Print and shaded views of the part. All mm, measured from the part's lowest x, y and z. Give positions to 0.01 mm unless a question says otherwise; leave off trailing zeros. Order: outer loops, then holes, each group sorted by start corner. A loop starts at its lowest first (then second) coordinate and runs counter-clockwise, first axis right, second up. Notation, with made-up numbers: (42.5, 31) - (86.5, 31) arc R15 ccw to (86.5, 54) - close; hole circle Ø7 at (82.25, -25.5). An arc over 180 degrees is marked (long way). Answer in a Markdown table with one row per item.
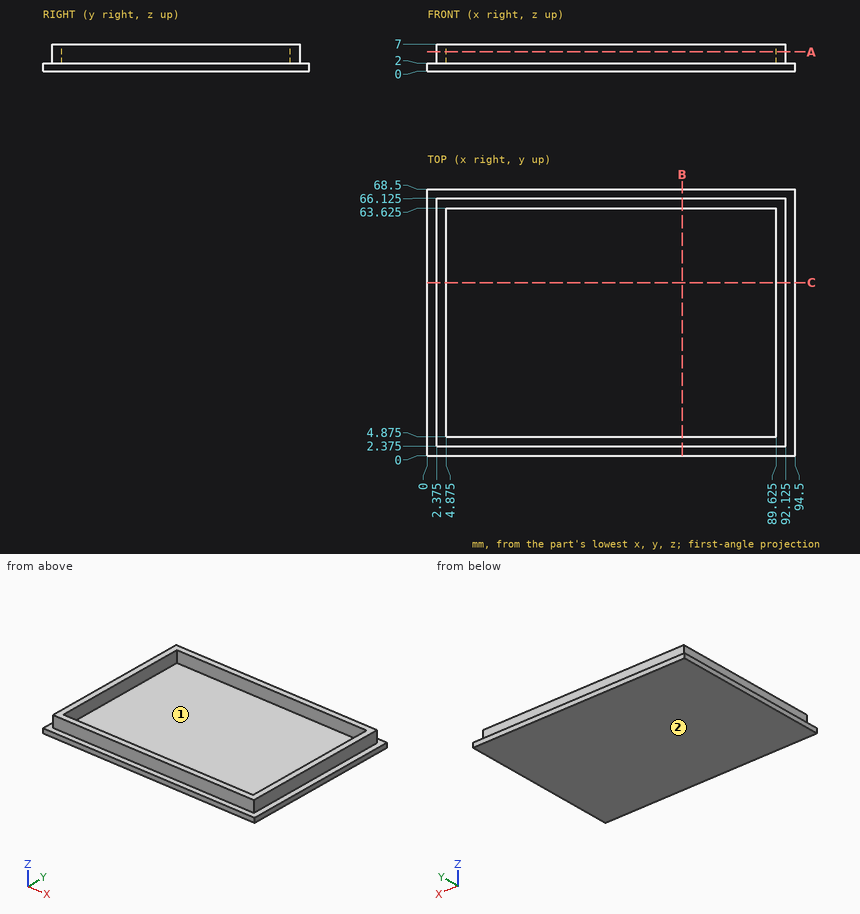
1. Cut at C-C on y = 44.5. Write the cut outline in (x, z) (3 decimals).
Check result:
| item | result |
|---|---|
| outline | (0, 0) - (94.5, 0) - (94.5, 2) - (92.125, 2) - (92.125, 7) - (89.625, 7) - (89.625, 2) - (4.875, 2) - (4.875, 7) - (2.375, 7) - (2.375, 2) - (0, 2) - close |
2. Two-plate mould, pull along Y, no slides. Class the marked faces 1 and 2: +Y half, -Y half, draft (parallel to the pull), parting line (faces both ways), or undercut.
Check result:
| item | result |
|---|---|
| face 1 | undercut |
| face 2 | draft |
3. Probe line 1 (X direction, y = 25.5, z = 4.5) (3 decimals); line 2 (Y direction, x = 45.5, z = 6.5) (3 decimals); line 3 (Z direction, x = 83.5, y = 54.5). List the from-to ranges inside material, lowest first.
Check result:
| item | result |
|---|---|
| line 1 | x = 2.375 to 4.875, 89.625 to 92.125 |
| line 2 | y = 2.375 to 4.875, 63.625 to 66.125 |
| line 3 | z = 0 to 2 |
4. Cut at B-B on x = 65.5. Write the cut outline in (y, z) (3 decimals).
Check result:
| item | result |
|---|---|
| outline | (0, 0) - (68.5, 0) - (68.5, 2) - (66.125, 2) - (66.125, 7) - (63.625, 7) - (63.625, 2) - (4.875, 2) - (4.875, 7) - (2.375, 7) - (2.375, 2) - (0, 2) - close |
5. Drop flat-ended pins along their axis: P1, Ø1.5, axis at x = 45.5, z = 5, coming from the +Y side (3 decimals); P2, Ø2.5, axis at x = 60, z = 4, coming from the -Y side (3 decimals); P3, Ø10, axis at x = 11, y = 43.5, coming from the +Z side. Give the stop position or say it passes through.
Check result:
| item | result |
|---|---|
| P1 | stops at y = 66.125 |
| P2 | stops at y = 2.375 |
| P3 | stops at z = 2 |
6. Cut at A-A on z = 5. Write the cut outline in (x, y) (3 decimals).
Check result:
| item | result |
|---|---|
| outline | (2.375, 2.375) - (92.125, 2.375) - (92.125, 66.125) - (2.375, 66.125) - close; hole (4.875, 4.875) - (89.625, 4.875) - (89.625, 63.625) - (4.875, 63.625) - close |
